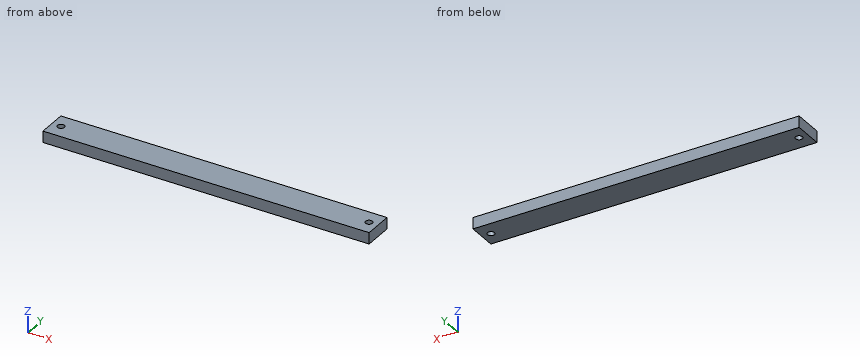
```python
from build123d import *

# Parameters (mm, degrees)
SKETCH1_W               = 717
SKETCH1_H               = 64.740437158
BOSS_EXTRUDE1_DEPTH     = 25
CUT_EXTRUDE1_DEPTH      = 361.825554875
CUT_EXTRUDE1_DEPTH_BACK = 361.825554875
SKETCH2_R               = 7.5


with BuildPart() as part:
    # Sketch1 → Boss-Extrude1 (new body)
    with BuildSketch(Plane.XY):
        Rectangle(SKETCH1_W, SKETCH1_H)
    extrude(amount=BOSS_EXTRUDE1_DEPTH)

    # Sketch2 → Cut-Extrude1 (cut, two sides: drawn at the far end of the back side and taken through both)
    with BuildSketch(Plane(origin=(0, 0, 0), x_dir=(-1, 0, 0), z_dir=(0, 0, -1)).offset(-CUT_EXTRUDE1_DEPTH_BACK)):
        with Locations((-338.5, 0)):
            Circle(SKETCH2_R)
        with Locations((338.5, 0)):
            Circle(SKETCH2_R)
    extrude(amount=CUT_EXTRUDE1_DEPTH + CUT_EXTRUDE1_DEPTH_BACK, mode=Mode.SUBTRACT)


solid = part.part
```
Part model, mm, in its own coordinate system. Give positions to 0.01 mm unless a question says otherwise; leave off trailing zeros. Order: outer loops, then holes, each group sorted by start corner. A loop starts at its lowest first (then second) coordinate and runs counter-clockwise, first axis right, second up. Notation, with made-up numbers: (19, 78) - (75, 78) arc R5 cw to (75, 83) - close; hole circle Ø8 at (-31, -38). An arc over 180 degrees is marked (long way). Use one line per item in the form item = value.
Item 1: Probe probe 1 along X at (y, z) = (0, 7); probe 2 along Y at (x, z) = (338.5, 17); probe 3 along X at (y, z) = (4, 16.5). List the from-to ranges inside material, lowest first. Write a range as from..to.
Solution:
probe_1 = -358.5..-346, -331..331, 346..358.5
probe_2 = -32.37..-7.5, 7.5..32.37
probe_3 = -358.5..-344.84, -332.16..332.16, 344.84..358.5
Item 2: Slice it at B-B on y = 0. Give the cut face in (x, z).
Solution:
outline = (-358.5, 0) - (-346, 0) - (-346, 25) - (-358.5, 25) - close; (-331, 0) - (331, 0) - (331, 25) - (-331, 25) - close; (346, 0) - (358.5, 0) - (358.5, 25) - (346, 25) - close
Item 3: Slice it at A-A on x = 338.5. Give the cut face in (y, z), and give its area (3 significant figures).
Solution:
outline = (-32.37, 0) - (-7.5, 0) - (-7.5, 25) - (-32.37, 25) - close; (7.5, 0) - (32.37, 0) - (32.37, 25) - (7.5, 25) - close
area = 1,240 mm2
Item 4: Pin check, flat tip, straight feed: pin 1 Ø13.5 at (x, y) = (338.5, 0) entering from -Z. Stop position of the tip, or through.
Solution:
pin_1 = through
